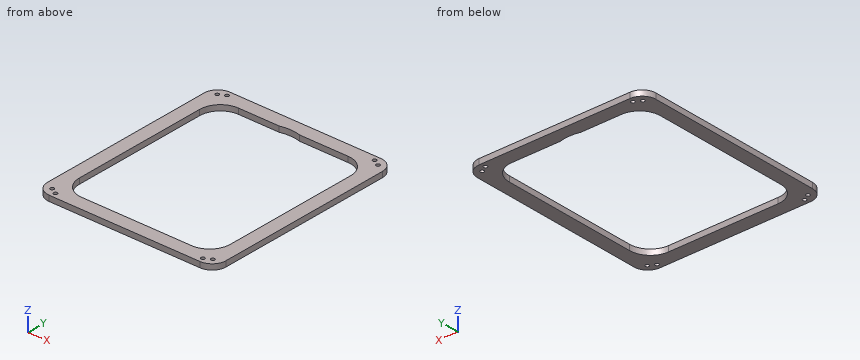
from build123d import *

# Parameters (mm, degrees)
F1_DEPTH = 5.08
F3_D     = 3.4544
F5_D     = 3.429
F6_R     = 36.195
F7_DEPTH = 5.081


with BuildPart() as f1:
    # F0 (on Top) → F1 (new body)
    with BuildSketch(Plane.XY):
        with BuildLine():
            ThreePointArc((0, 12.7), (3.7197438789, 3.7197438789), (12.7, 0))
            Line((12.7, 0), (152.4, 0))
            ThreePointArc((152.4, 0), (161.3802561211, 3.7197438789), (165.1, 12.7))
            Line((165.1, 12.7), (165.1, 177.8))
            ThreePointArc((165.1, 177.8), (161.3802561211, 186.7802561211), (152.4, 190.5))
            Line((152.4, 190.5), (12.7, 190.5))
            ThreePointArc((12.7, 190.5), (3.7197438789, 186.7802561211), (0, 177.8))
            Line((0, 177.8), (0, 12.7))
        make_face()
        with BuildLine():
            ThreePointArc((12.7, 158.75), (18.2796158184, 172.2203841816), (31.75, 177.8))
            Line((31.75, 177.8), (133.35, 177.8))
            ThreePointArc((133.35, 177.8), (146.8203841816, 172.2203841816), (152.4, 158.75))
            Line((152.4, 158.75), (152.4, 31.75))
            ThreePointArc((152.4, 31.75), (146.8203841816, 18.2796158184), (133.35, 12.7))
            Line((133.35, 12.7), (31.75, 12.7))
            ThreePointArc((31.75, 12.7), (18.2796158184, 18.2796158184), (12.7, 31.75))
            Line((12.7, 31.75), (12.7, 158.75))
        make_face(mode=Mode.SUBTRACT)
    extrude(amount=F1_DEPTH)

    # F3 (through all)
    with Locations(Plane(origin=(0, 0, 0), x_dir=(1, 0, 0), z_dir=(0, 0, -1))):
        with Locations((8.2098719395, -182.2901280605), (156.8901280605, -182.2901280605), (156.8901280605, -8.2098719395), (8.2098719395, -8.2098719395)):
            Hole(F3_D / 2)

    # F5 (through all)
    with Locations(Plane.XY.offset(5.08)):
        with Locations((14.3002, 185.7248), (150.7998, 185.7248), (14.3002, 4.7752), (150.7998, 4.7752)):
            Hole(F5_D / 2)

    # F6 (on face) → F7 (cut, through all)
    with BuildSketch(Plane.XY.offset(5.08)):
        with Locations((79.0035873652, 142.875)):
            Circle(F6_R)
    extrude(amount=-F7_DEPTH, mode=Mode.SUBTRACT)


solid = f1.part
Verification items for the finished model (mm, model axes). Give positions to 0.01 mm unless a question says otherwise; leave off trailing zeros. Write each loop counter-clockwise with the first axis right and the second up, starting at its lowest first coordinate (ties: lowest second). Pieces come first, ordered by that corner, then holes. Notation, with made-up numbers: M 54,28.5 L 73,28.5 A22 ccw 73,62.5 Z; hole C -13,17.5 d5. An arc over 180 degrees is marked long. Put each result on its own line as item: value. Start each with the question number.
1. Section check C-C (z = 1.4). Give the number of separate pieces and of enclosed holes in the cut face, and give its area (3 significant figures).
2. Section check B-B (x = 140.5). Record the cut outline in (y, z), and give its area (3 significant figures).
3. Scan lines: line 1 along Y through (x, z) = (46, 4.55); line 2 along X through (y, z) = (68, 2.35); line 3 along Y through (x, z) = (78, 4.1). Record each from-to range of solid material in increasing order. Write a range as [from, to].
4. Go/stop test with a flat-tipped pin: pin 1 Ø2 at (x, y) = (8.21, 182.29) entering from -Z. Record where the tip stops, or that it passes through.
5. Section check A-A (y = 39.5). Record the cut outline in (x, z), and give its area (3 significant figures).
Answer list:
1. separate pieces: 1
1. enclosed holes: 9
1. area: 8,470 mm2
2. outline: M 0,0 L 14.09,0 L 14.09,5.08 L 0,5.08 Z; M 176.41,0 L 190.5,0 L 190.5,5.08 L 176.41,5.08 Z
2. area: 143 mm2
3. line 1: [0, 12.7], [177.8, 190.5]
3. line 2: [0, 12.7], [152.4, 165.1]
3. line 3: [0, 12.7], [179.06, 190.5]
4. pin 1: through
5. outline: M 0,0 L 12.7,0 L 12.7,5.08 L 0,5.08 Z; M 152.4,0 L 165.1,0 L 165.1,5.08 L 152.4,5.08 Z
5. area: 129 mm2
